Geometry: see drawing. Coordinates: mm, zero at the bounding-box minimum. A direction names the side the tool comes from. Coordinates: 2 decimals unless noted, no trailing zeros. Loops run counter-clockwise (first coordinate to the right, second up) from the corner with the lowest first, then second, coordinate; pieces in that order, holes last. Notation, with made-up numbers: (20, 4.25) - (33, 4.25) arc R27 cw to (33, 37.25) - close; hole circle Ø7 at (-25, 3). An arc over 180 degrees is marked (long way). Write item = value, one per line. Start each with the question number.
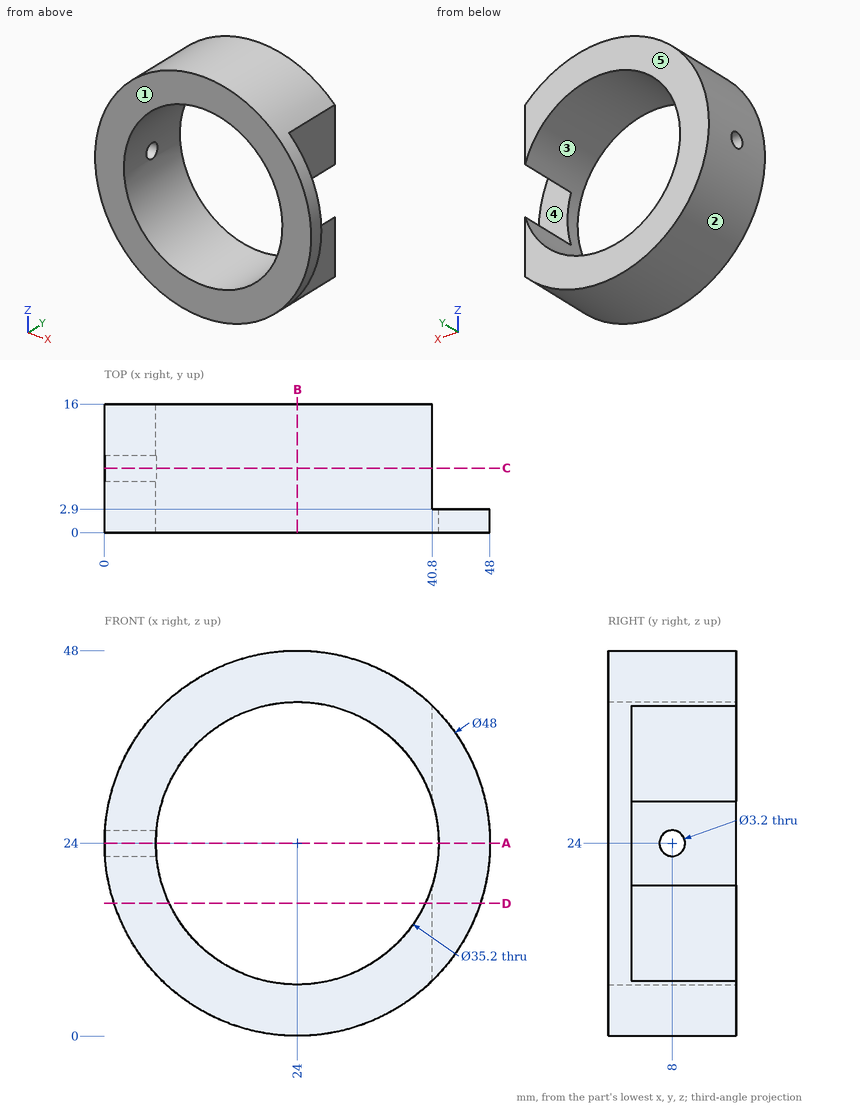
Item 1: Cut plane A-A (z = 24). Return the cut outline in (x, y), then the cut area to 3 significant figures.
Item 2: First-contact query: pin 1 (1 mm diameter, centred on y = 11, z = 28.5, fed in from +X); pin 2 (2 mm diameter, centred on x = 21.5, y = 8.5, fed in from +Z); pin 3 (6 mm diameter, centred on y = 9, z = 13, fed in from +X). Flat tips, straight axial feed; report the tip coordinate or a pass-through.
Item 3: Cut plane D-D (z = 16.5). Return the cut outline in (x, y), then the cut area to 3 significant figures.
Item 4: Material intervals for L1, parallel to Y at x = 2.25, z = 24; L2, parallel to X at y = 4.75, z = 10; L3, parallel to Z at x = 10, y = 13.25, sorted ascending. Write a range as [from, to].
Item 5: Reachability of the marked faces 4 and 5 from +Z, -Z, +X, -X, +Y, -Y: full face, straight path, thin tool, end or side. Return the list, or none.
Item 6: Cut plane C-C (y = 8). Return the cut outline in (x, z).
Item 7: Cut plane B-B (x = 24). Return the cut outline in (y, z).
Item 8: Draft query along Z for the marked faces 1, 2 and 3. Return one class per face: released by +Z, released by -Z, zero draft, split by the parting line, or undercut.
Responses:
q1.outline = (0, 0) - (6.4, 0) - (6.4, 6.4) - (0, 6.4) - close; (0, 9.6) - (6.4, 9.6) - (6.4, 16) - (0, 16) - close; (41.6, 0) - (48, 0) - (48, 2.9) - (41.6, 2.9) - close
q1.area = 100 mm2
q2.pin_1 = 7.13
q2.pin_2 = 47.95
q2.pin_3 = 40.8
q3.outline = (1.2, 0) - (8.08, 0) - (8.08, 16) - (1.2, 16) - close; (39.92, 0) - (46.8, 0) - (46.8, 2.9) - (40.8, 2.9) - (40.8, 16) - (39.92, 16) - close
q3.area = 141 mm2
q4.L1 = [0, 6.4], [9.6, 16]
q4.L2 = [4.51, 13.33], [34.67, 40.8]
q4.L3 = [4.51, 13.33], [34.67, 43.49]
q5.face_4 = +Z, -Z, +X, +Y
q5.face_5 = +Z, -Z, +X, -X, +Y
q6.outline = (0.05, 22.4) arc R24 ccw to (40.8, 6.86) - (40.8, 18.75) arc R17.6 cw to (6.47, 22.4) - close; (0.05, 25.6) - (6.47, 25.6) arc R17.6 cw to (40.8, 29.25) - (40.8, 41.14) arc R24 ccw to start
q7.outline = (0, 0) - (16, 0) - (16, 6.4) - (0, 6.4) - close; (0, 41.6) - (16, 41.6) - (16, 48) - (0, 48) - close
q8.face_1 = zero draft
q8.face_2 = split by the parting line
q8.face_3 = undercut
